```python
from build123d import *

# Parameters (mm, degrees)
F1_DEPTH  = 8
F3_DEPTH  = 621.7
F4_DEPTH  = 5.5
F7_DEPTH  = 5.5
F9_DEPTH  = 5.5
F11_DEPTH = 5.5
F13_DEPTH = 5.5
F15_DEPTH = 5.5
F17_DEPTH = 308.2
F18_DEPTH = 24
F20_DEPTH = 244.2
F21_DEPTH = 30.35
F22_R     = 2.5
F23_DEPTH = 0.5
F24_R     = 2.5
F25_DEPTH = 0.5
F26_R     = 2.5
F27_DEPTH = 0.5
F28_R     = 2.5
F29_DEPTH = 0.5
F30_W     = 14.1428571429
F30_H     = 18
F30_W_2   = 4.1785714286
F30_H_2   = 6.1071428571
F31_DEPTH = 0.5
F32_DEPTH = 25
F34_DEPTH = 8


# Not quite as in the source:
# - a feature of the source that left no trace in its solid (it failed there, or was rolled back) is left out


with BuildPart() as f1:
    # F0 (on Top) → F1 (new body)
    with BuildSketch(Plane.XY):
        Polygon((-327.3, 108.1424002851), (-327.3, -140.8575997149), (-102.6, -140.8575997149), (-102.6, -170.8575997149), (0, -170.8575997149), (0, -140.8575997149), (288.9, -140.8575997149), (288.9, 108.1424002851), (0, 108.1424002851), (0, 138.1424002851), (-102.6, 128.6424002851), (-102.6, 108.1424002851), align=None)
    extrude(amount=F1_DEPTH)

    # F2 (on face) → F3 (join)
    with BuildSketch(Plane.YZ.offset(288.9)):
        Polygon((-16.3575997149, 51.4532495908), (-146.3575997149, 8), (-140.8575997149, 8), (108.1424002851, 8), (113.6424002851, 8), align=None)
    extrude(amount=-F3_DEPTH)

    # F2 (on face) → F4 (join)
    with BuildSketch(Plane.YZ.offset(288.9)):
        Polygon((-16.3575997149, 51.4532495908), (-146.3575997149, 8), (113.6424002851, 8), align=None)
    extrude(amount=F4_DEPTH)

    # F5 (on face) → F7 (join)
    with BuildSketch(Plane.XZ.offset(170.8575997149)):
        Polygon((-51.3, 62.75), (-108.1, 8), (5.5, 8), align=None)
    extrude(amount=F7_DEPTH)

    # F8 (on face) → F9 (cut)
    with BuildSketch(Plane(origin=(-13.187163576, 142.4213666207, 0), x_dir=(-0.9957406741, -0.0921982106, 0), z_dir=(-0.0921982106, 0.9957406741, 0))):
        Polygon((91.8565413643, 4.3927081219), (38.2758658123, 55.8195932448), (-15.3048097397, 4.3927081219), align=None)
    extrude(amount=-F9_DEPTH, mode=Mode.SUBTRACT)

    # F10 (on face) → F11 (cut)
    with BuildSketch(Plane(origin=(-332.8, 0, 0), x_dir=(0, -1, 0), z_dir=(-1, 0, 0))):
        Polygon((144.6140170728, 2.7836871671), (16.3575997149, 45.6541342062), (-111.8988176431, 2.7836871671), align=None)
    extrude(amount=-F11_DEPTH, mode=Mode.SUBTRACT)

    # F12 (on face) → F13 (cut)
    with BuildSketch(Plane.YZ.offset(294.4)):
        Polygon((111.8988176431, 2.7836871671), (-16.3575997149, 45.6541342062), (-144.6140170728, 2.7836871671), align=None)
    extrude(amount=-F13_DEPTH, mode=Mode.SUBTRACT)

    # F14 (on face) → F15 (cut)
    with BuildSketch(Plane.XZ.offset(176.3575997149)):
        Polygon((1.6830285492, 4.0401099834), (-51.3, 55.1108989459), (-104.2830285492, 4.0401099834), align=None)
    extrude(amount=-F15_DEPTH, mode=Mode.SUBTRACT)

    # F16 (on face) → F17 (join)
    with BuildSketch(Plane.YZ.offset(294.4)):
        Polygon((-37.9123742622, 48.4659791319), (-36.6443145321, 44.6722981882), (-16.3575997149, 51.4532495908), (3.9291151024, 44.6722981882), (5.1971748325, 48.4659791319), (-16.3575997149, 55.670786811), align=None)
    extrude(amount=-F17_DEPTH)

    # F16 (on face) → F18 (cut)
    with BuildSketch(Plane.YZ.offset(294.4)):
        Polygon((-37.9123742622, 48.4659791319), (-36.6443145321, 44.6722981882), (-16.3575997149, 51.4532495908), (3.9291151024, 44.6722981882), (5.1971748325, 48.4659791319), (-16.3575997149, 55.670786811), align=None)
    extrude(amount=-F18_DEPTH, mode=Mode.SUBTRACT)

    # F19 (on face) → F20 (join)
    with BuildSketch(Plane(origin=(-332.8, 0, 0), x_dir=(0, -1, 0), z_dir=(-1, 0, 0))):
        Polygon((-5.1971748325, 48.4659791319), (-3.9291151024, 44.6722981882), (16.3575997149, 51.4532495908), (36.6443145321, 44.6722981882), (37.9123742622, 48.4659791319), (16.3575997149, 55.670786811), align=None)
    extrude(amount=-F20_DEPTH)

    # F19 (on face) → F21 (cut)
    with BuildSketch(Plane(origin=(-332.8, 0, 0), x_dir=(0, -1, 0), z_dir=(-1, 0, 0))):
        Polygon((-5.1971748325, 48.4659791319), (-3.9291151024, 44.6722981882), (16.3575997149, 51.4532495908), (36.6443145321, 44.6722981882), (37.9123742622, 48.4659791319), (16.3575997149, 55.670786811), align=None)
    extrude(amount=-F21_DEPTH, mode=Mode.SUBTRACT)

    # F22 (on face) → F23 (cut)
    with BuildSketch(Plane(origin=(-327.3, 0, 0), x_dir=(0, -1, 0), z_dir=(-1, 0, 0))):
        with Locations((8.3575997149, 35)):
            Circle(F22_R)
        with Locations((24.3575997149, 35)):
            Circle(F22_R)
    extrude(amount=-F23_DEPTH, mode=Mode.SUBTRACT)

    # F24 (on face) → F25 (cut)
    with BuildSketch(Plane.YZ.offset(288.9)):
        with Locations((-24.3575997149, 35)):
            Circle(F24_R)
        with Locations((-8.3575997149, 35)):
            Circle(F24_R)
    extrude(amount=-F25_DEPTH, mode=Mode.SUBTRACT)

    # F26 (on face) → F27 (cut)
    with BuildSketch(Plane.XZ.offset(170.8575997149)):
        with Locations((-59.3, 35)):
            Circle(F26_R)
        with Locations((-43.3, 35)):
            Circle(F26_R)
    extrude(amount=-F27_DEPTH, mode=Mode.SUBTRACT)

    # F28 (on face) → F29 (cut)
    with BuildSketch(Plane(origin=(-12.6822332802, 136.9681194259, 0), x_dir=(-0.9957406741, -0.0921982106, 0), z_dir=(-0.0921982106, 0.9957406741, 0))):
        with Locations((30.7829559704, 35)):
            Circle(F28_R)
        with Locations((46.7829559704, 35)):
            Circle(F28_R)
    extrude(amount=-F29_DEPTH, mode=Mode.SUBTRACT)

    # F30 (on face) → F31 (cut)
    with BuildSketch(Plane.YZ.offset(288.9)):
        with Locations((-16.3575997149, 14)):
            Rectangle(F30_W, F30_H)
        with Locations((-19.4111711434, 9.9821428571)):
            Rectangle(F30_W_2, F30_H_2, mode=Mode.SUBTRACT)
        with Locations((-13.3040282863, 9.9821428571)):
            Rectangle(F30_W_2, F30_H_2, mode=Mode.SUBTRACT)
        with Locations((-19.4111711434, 18.0178571429)):
            Rectangle(F30_W_2, F30_H_2, mode=Mode.SUBTRACT)
        with Locations((-13.3040282863, 18.0178571429)):
            Rectangle(F30_W_2, F30_H_2, mode=Mode.SUBTRACT)
        with Locations((18.6424002851, 14)):
            Rectangle(F30_W, F30_H)
        with Locations((15.5888288566, 9.9821428571)):
            Rectangle(F30_W_2, F30_H_2, mode=Mode.SUBTRACT)
        with Locations((21.6959717137, 9.9821428571)):
            Rectangle(F30_W_2, F30_H_2, mode=Mode.SUBTRACT)
        with Locations((15.5888288566, 18.0178571429)):
            Rectangle(F30_W_2, F30_H_2, mode=Mode.SUBTRACT)
        with Locations((21.6959717137, 18.0178571429)):
            Rectangle(F30_W_2, F30_H_2, mode=Mode.SUBTRACT)
        with Locations((-51.3575997149, 14)):
            Rectangle(F30_W, F30_H)
        with Locations((-54.4111711434, 9.9821428571)):
            Rectangle(F30_W_2, F30_H_2, mode=Mode.SUBTRACT)
        with Locations((-48.3040282863, 9.9821428571)):
            Rectangle(F30_W_2, F30_H_2, mode=Mode.SUBTRACT)
        with Locations((-54.4111711434, 18.0178571429)):
            Rectangle(F30_W_2, F30_H_2, mode=Mode.SUBTRACT)
        with Locations((-48.3040282863, 18.0178571429)):
            Rectangle(F30_W_2, F30_H_2, mode=Mode.SUBTRACT)
    extrude(amount=-F31_DEPTH, mode=Mode.SUBTRACT)


with BuildPart() as f32:
    # F32 (new): a face of the model
    f32_faces = [f1.part.faces().sort_by_distance(p)[0] for p in [
        (-327.3, -16.3575997149, 15.1372563079),
    ]]
    extrude(f32_faces, amount=F32_DEPTH)

    # F34 (cut): a face of the model
    f34_faces = [f32.faces().sort_by_distance(p)[0] for p in [
        (-339.8, -16.3575997149, 0),
    ]]
    extrude(f34_faces, amount=-F34_DEPTH, mode=Mode.SUBTRACT)


solid = f32.part
```
Geometry: final body of the model. Coordinates: model frame, mm. Round coordinates to 2 decimals unless told otherwise and drop trailing zeros. Loops run counter-clockwise (first coordinate to the right, second up) from the corner with the lowest first, then second, coordinate; pieces in that order, holes last.
Item 1: Section A-A, the plane x = -338.5. Output: boundary loops of the cut face in (y, z).
Checked values:
outline: (-129.01, 8) - (96.29, 8) - (-16.36, 45.65) - close; hole circle Ø5 at (-24.36, 35); hole circle Ø5 at (-8.36, 35)
Item 2: Mould query, pull axis Z, two halves, no side actions, for faces 1 (the flat face through (-339.62, 39.18, 27.09)), 2 (the cylindrical face through (-339.625, -10.742, 35.751)), 3 (the flat face through (-352.3, -15, 22)). Classes: released by +Z, released by -Z, zero draft, split by the parting line, or undercut.
Checked values:
face 1: released by +Z
face 2: undercut
face 3: zero draft
Item 3: Section C-C, the plane y = -34. Output: boundary loops of the cut face in (x, z), plus the area to 3 significant figures.
Checked values:
outline: (-352.3, 8) - (-327.3, 8) - (-327.3, 39.76) - (-352.3, 39.76) - close
area: 794 mm2
Item 4: Section D-D, the plane z = 16. Output: boundary loops of the cut face in (x, y).
Checked values:
outline: (-352.3, -105.07) - (-327.3, -105.07) - (-327.3, 72.36) - (-352.3, 72.36) - close
Item 5: Section B-B, the plane z = 35. Output: boundary loops of the cut face in (x, y).
Checked values:
outline: (-352.3, -48.23) - (-327.3, -48.23) - (-327.3, -26.86) - (-352.3, -26.86) - close; (-352.3, -21.86) - (-327.3, -21.86) - (-327.3, -10.86) - (-352.3, -10.86) - close; (-352.3, -5.86) - (-327.3, -5.86) - (-327.3, 15.52) - (-352.3, 15.52) - close
Item 6: Line query: L1, parallel to Z at x = -329.75, y = -98; L2, parallel to Z at x = -342.25, y = 0. Output: solid intervals per line, ascending.
Checked values:
L1: z = 8 to 18.36
L2: z = 8 to 40.19
Item 7: Contact query for flat-ended pins moving along their axis: P1, Ø12, axis at x = -337, y = -95, coming from the +Z side; P2, Ø12, axis at x = -348.5, y = 54, coming from the +Z side; P3, Ø10, axis at y = -81, z = 27, coming from the -X side. Output: stop coordinate, or through.
Checked values:
P1: stops at z = 21.37
P2: stops at z = 24.14
P3: stops at x = -352.3
